Source: three-view drawing plus pictorial views. Frame: mm from the lowest corner of the part. A direction names the side the tool comes from. Give positions to 0.01 mm unless a question says otherwise; leave off trailing zeros. Loops run counter-clockwise (first coordinate to the right, second up) from the corner with the lowest first, then second, coordinate; pieces in that order, holes last. Notation, with made-up numbers: M 23,88.5 L 52,88.5 A20 cw 52,99.5 Z; hole C -13.5,-38 d1. An arc over 180 degrees is marked long. Write item = value, one per line.
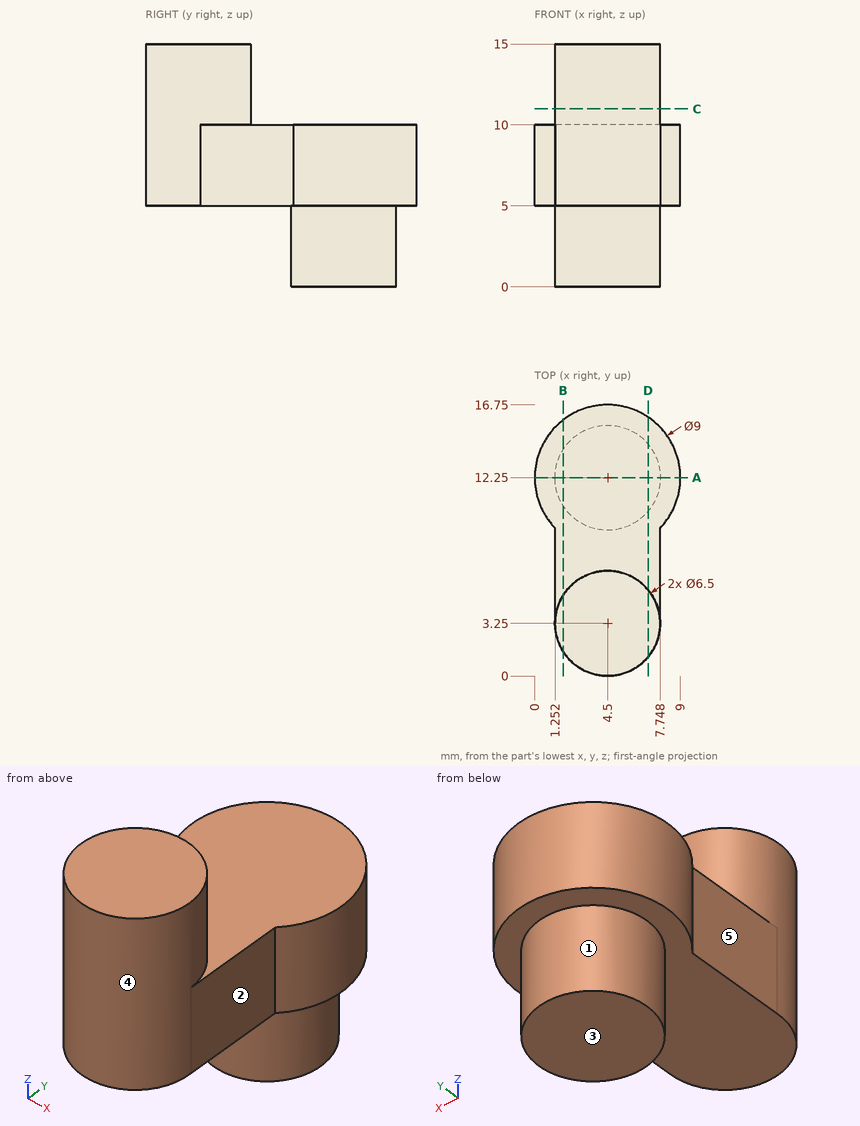
1. Cut plane D-D, the plane x = 7. Return the cut outline in (y, z), then the cut area to 3 significant figures.
Derived:
outline = M 1.17,5 L 10.17,5 L 10.17,0 L 14.33,0 L 14.33,5 L 15.99,5 L 15.99,10 L 5.33,10 L 5.33,15 L 1.17,15 Z
area = 116 mm²
2. Material intervals for probe 1 along Z at (x, y) = (5.25, 2.5); probe 2 along Z at (x, y) = (3.5, 15); probe 3 along X at (y, z) = (3.25, 7.75), sorted ascending. Write a range as from..to.
Derived:
probe_1 = 5..15
probe_2 = 0..10
probe_3 = 1.25..7.75
3. Cut plane A-A, the plane y = 12.25. Return the cut outline in (x, z).
Derived:
outline = M 0,5 L 1.25,5 L 1.25,0 L 7.75,0 L 7.75,5 L 9,5 L 9,10 L 0,10 Z
4. Cut plane B-B, the plane x = 1.75. Return the cut outline in (y, z).
Derived:
outline = M 1.52,5 L 10.52,5 L 10.52,0 L 13.98,0 L 13.98,5 L 15.81,5 L 15.81,10 L 4.98,10 L 4.98,15 L 1.52,15 Z
5. Cut plane C-C, the plane z = 11. Return the cut outline in (x, y), then the cut area to 3 significant figures.
Derived:
outline = C 4.5,3.25 d6.5
area = 33.2 mm²
6. Reachability of the marked faces 1, 2, 3, 4 and 5 from +Z, -Z, +X, -X, +Y, -Y: full face, straight path, thin tool, end or side. Return the list, or none.
Derived:
face_1 = -Z
face_2 = +Z, -Z, +X, -Y
face_3 = -Z, +X, -X, +Y, -Y
face_4 = +Z
face_5 = +Z, -Z, -X, -Y
7. First-contact query: pin 1 Ø5.5 at (y, z) = (5, 8.5) entering from -X; pin 2 Ø1 at (x, y) = (6, 3.5) entering from -Z; pin 3 Ø2.5 at (y, z) = (5, 7.5) entering from +X. Flat tips, straight axial feed; report the tip coordinate or a pass-through.
Derived:
pin_1 = 1.25
pin_2 = 5
pin_3 = 7.75
